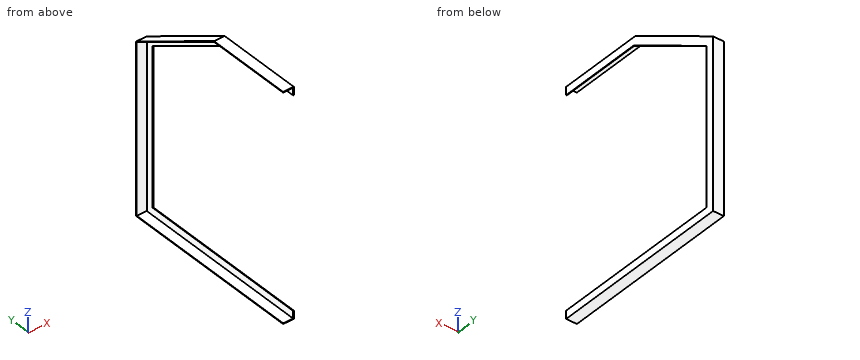
```python
from build123d import *

# Parameters (mm, degrees)
BOSS_EXTRUDE1_DEPTH = 3.175
BOSS_EXTRUDE2_DEPTH = 47.625


with BuildPart() as part:
    # Sketch1 → Boss-Extrude1 (new body)
    with BuildSketch(Plane(origin=(0, 0, 0), x_dir=(0, 0, -1), z_dir=(1, 0, 0))):
        Polygon((-495.3, 0), (-495.3, 396.191135768), (-247.43841167, 825.5), (495.3, 825.5), (495.3, 0), (533.4, 0), (533.4, 863.6), (-269.435456927, 863.6), (-533.4, 406.4), (-533.4, 0), align=None)
    extrude(amount=BOSS_EXTRUDE1_DEPTH)

    # Sketch2 → Boss-Extrude2 (add)
    with BuildSketch(Plane.ZY):
        Polygon((530.225, 0), (530.225, 405.549261314), (267.602369822, 860.425), (-530.225, 860.425), (-530.225, 0), (-533.4, 0), (-533.4, 863.6), (269.435456927, 863.6), (533.4, 406.4), (533.4, 0), align=None)
    extrude(amount=BOSS_EXTRUDE2_DEPTH)


solid = part.part
```
Input: part model. Units: mm. Frame: model coordinates. Round coordinates to 2 decimals unless told otherwise and drop trailing zeros. Loops run counter-clockwise (first coordinate to the right, second up) from the corner with the lowest first, then second, coordinate; pieces in that order, holes last. Notation, with made-up numbers: (-36.5, -25.5) -> (14.5, -25.5) arc R12 cw to (14.5, -20.5) -> close; hole circle Ø7 at (-33.5, 65.5). An arc over 180 degrees is marked (long way). Use one line per item in the form item = value. Start each with the question number.
Item 1: Section query B-B on x = -21. Return the cut outline in (y, z) (3 decimals), then the cut area to 3 significant figures.
Item 2: Section query D-D on y = 758. Return the cut outline in (x, z) (3 decimals), then the cut area to 3 significant figures.
Item 3: Material intervals for L1, parallel to Z at x = -29, y = 193 (3 decimals); L2, parallel to Y at x = -27.5, z = 164 (3 decimals); L3, parallel to Z at x = -33, y = 606.5 (3 decimals), sorted ascending. Write a range as from..to.
Item 4: Section query C-C on z = 154. Return the cut outline in (x, y) (3 decimals), then the cut area to 3 significant figures.
Item 5: Section query A-A on y = 57. Return the cut outline in (x, z) (3 decimals), then the cut area to 3 significant figures.
Item 6: Contact query for flat-ended pins moving along their axis: pin 1 Ø3 at (x, y) = (-24.5, 510.5) entering from +Z; pin 2 Ø5 at (x, z) = (-19.5, -15.5) entering from -Y (3 decimals); pin 3 Ø2.5 at (x, z) = (1.5, -169) entering from -Y. Output: stop coordinate, or through.
Ans:
q1.outline = (0, -533.4) -> (863.6, -533.4) -> (863.6, 269.435) -> (406.4, 533.4) -> (0, 533.4) -> (0, 530.225) -> (405.549, 530.225) -> (860.425, 267.602) -> (860.425, -530.225) -> (0, -530.225) -> close
q1.area = 8,240 mm^2
q2.outline = (-47.625, -533.4) -> (3.175, -533.4) -> (3.175, -495.3) -> (0, -495.3) -> (0, -530.225) -> (-47.625, -530.225) -> close; (-47.625, 326.737) -> (0, 326.737) -> (0, 286.41) -> (3.175, 286.41) -> (3.175, 330.404) -> (-47.625, 330.404) -> close
q2.area = 586 mm^2
q3.L1 = -533.4..-530.225, 530.225..533.4
q3.L2 = 860.425..863.6
q3.L3 = -533.4..-530.225, 414.206..417.872
q4.outline = (-47.625, 860.425) -> (0, 860.425) -> (0, 825.5) -> (3.175, 825.5) -> (3.175, 863.6) -> (-47.625, 863.6) -> close
q4.area = 272 mm^2
q5.outline = (-47.625, -533.4) -> (3.175, -533.4) -> (3.175, -495.3) -> (0, -495.3) -> (0, -530.225) -> (-47.625, -530.225) -> close; (-47.625, 530.225) -> (0, 530.225) -> (0, 495.3) -> (3.175, 495.3) -> (3.175, 533.4) -> (-47.625, 533.4) -> close
q5.area = 544 mm^2
q6.pin_1 = 474.16
q6.pin_2 = 860.425
q6.pin_3 = 825.5
